Source: CAD feature listing. Evaluate the final solid. Frame: model axes, mm. A direction names the side the tool comes from. Give positions to 0.01 mm unless a question says otherwise; leave off trailing zeros. Write each loop counter-clockwise with the first axis right and the second up, starting at its lowest first coordinate (ties: lowest second). Pieces come first, ordered by that corner, then holes. Notation, with made-up numbers: M 57,-13 L 63,-13 A20 cw 63,26 Z; hole C 47,58 d5. An arc over 180 degrees is marked long. Return JSON: item names as keys, results as strings.
```python
from build123d import *

# Parameters (mm, degrees)
SKETCH_1_R      = 1.5
SKETCH_1_R_2    = 8
SKETCH_1_R_3    = 2
EXTRUDE_1_DEPTH = 2
FILLET_1_R      = 5


with BuildPart() as part:
    # 草图1 → 凸台-拉伸1 (new body)
    with BuildSketch(Plane.XY):
        Polygon((20, -19), (-4, -19), (-4, -32), (-16, -43), (-16, -61), (-4, -70), (-4, -77), (20, -77), (20, -70), (32, -61), (32, -43), (20, -32), align=None)
        with Locations((8, -65.75)):
            Circle(SKETCH_1_R, mode=Mode.SUBTRACT)
        with Locations((8, -38.25)):
            Circle(SKETCH_1_R_2, mode=Mode.SUBTRACT)
        with Locations((3, -72)):
            Circle(SKETCH_1_R_3, mode=Mode.SUBTRACT)
        with Locations((13, -72)):
            Circle(SKETCH_1_R_3, mode=Mode.SUBTRACT)
        with Locations((-12, -48)):
            Circle(SKETCH_1_R_3, mode=Mode.SUBTRACT)
        with Locations((-12, -56)):
            Circle(SKETCH_1_R_3, mode=Mode.SUBTRACT)
        with Locations(Location((28, -57, 0), (0, 0, 180))):
            Circle(SKETCH_1_R_3, mode=Mode.SUBTRACT)
        with Locations(Location((28, -47, 0), (0, 0, 180))):
            Circle(SKETCH_1_R_3, mode=Mode.SUBTRACT)
        with Locations((3, -24)):
            Circle(SKETCH_1_R_3, mode=Mode.SUBTRACT)
        with Locations((13, -24)):
            Circle(SKETCH_1_R_3, mode=Mode.SUBTRACT)
        with BuildLine():
            Line((4, -55), (12, -55))
            ThreePointArc((12, -55), (15.5, -58.5), (12, -62))
            Line((12, -62), (4, -62))
            ThreePointArc((4, -62), (0.5, -58.5), (4, -55))
        make_face(mode=Mode.SUBTRACT)
    extrude(amount=EXTRUDE_1_DEPTH)

    # 圆角1
    fillet_1_edges = [part.edges().sort_by_distance(p)[0] for p in [
        (32, -43, 1),
        (20, -19, 1),
        (-4, -19, 1),
        (-16, -43, 1),
        (-16, -61, 1),
        (-4, -77, 1),
        (20, -77, 1),
        (32, -61, 1),
    ]]
    fillet(fillet_1_edges, radius=FILLET_1_R)


solid = part.part
```
1) Contact query for a flat-ended pin moving along its axis: pin 1 Ø1 at (y, z) = (-30, 0.5) entering from +X. Output: stop coordinate, or through.
Numbers:
{"pin 1": "stops at x = 20"}
2) Set-up query: faces 1 (the face through (20, -28, 1)), 2 (the face through (-4, -71, 1)), 3 (the face through (-4, -28, 1)), 4 (the face through (8, -77, 1)), 5 (the face through (20, -71, 1)). Return all of +Z, -Z, +X, -X, +Y, -Y with unobstructed straight access to the full face (end or side cutting, diameter ignored); none if empty.
Numbers:
{"face 1": "+Z, -Z, +X, +Y", "face 2": "+Z, -Z, -X, -Y", "face 3": "+Z, -Z, -X, +Y", "face 4": "+Z, -Z, +X, -X, -Y", "face 5": "+Z, -Z, +X, -Y"}
3) Cut plane C-C, the plane y = -35.5. Return the cut outline in (x, z), then the cut area to 3 significant figures.
Numbers:
{"outline": "M -7.82,0 L 0.49,0 L 0.49,2 L -7.82,2 Z; M 15.51,0 L 23.82,0 L 23.82,2 L 15.51,2 Z", "area": "33.2 mm²"}
4) Cut plane B-B, the plane z = 0.45. Give the number of separate pieces and of enclosed holes in the cut face, then the cut area to 3 significant figures.
Numbers:
{"separate pieces": "1", "enclosed holes": "11", "area": "1,640 mm²"}
5) Cut plane D-D, the plane y = -57. Return the cut outline in (x, z).
Numbers:
{"outline": "M -16,0 L -13.73,0 L -13.73,2 L -16,2 Z; M -10.27,0 L 0.84,0 L 0.84,2 L -10.27,2 Z; M 15.16,0 L 26,0 L 26,2 L 15.16,2 Z; M 30,0 L 32,0 L 32,2 L 30,2 Z"}
6) Cut plane A-A, the plane x = 8. Return the cut outline in (y, z).
Numbers:
{"outline": "M -77,0 L -67.25,0 L -67.25,2 L -77,2 Z; M -64.25,0 L -62,0 L -62,2 L -64.25,2 Z; M -55,0 L -46.25,0 L -46.25,2 L -55,2 Z; M -30.25,0 L -19,0 L -19,2 L -30.25,2 Z"}
7) Draft query along Y for faces 6 (the face through (8, -48, 0)), 7 (the face through (19, -75, 1)), 8 (the face through (-12, -50, 1)). Return one class per face: released by +Y, released by -Y, zero draft, split by the parting line, or undercut.
Numbers:
{"face 6": "zero draft", "face 7": "released by -Y", "face 8": "undercut"}
8) Line query: line 1 (X direction, y = -71, z = 1.25); line 2 (X direction, y = -47, z = 0.95); line 3 (Y direction, x = 10.5, z = 0.5). Output: solid intervals per line, ascending. Write a range as [from, to].
Numbers:
{"line 1": "x = [-4, 1.27], [4.73, 11.27], [14.73, 20]", "line 2": "x = [-16, -13.73], [-10.27, 26], [30, 32]", "line 3": "y = [-77, -62], [-55, -45.85], [-30.65, -19]"}
